CAD build for the part. Positions are in the model's coordinates, mm. Coordinates: 2 decimals unless noted, no trailing zeros. Loops run counter-clockwise (first coordinate to the right, second up) from the corner with the lowest first, then second, coordinate; pieces in that order, holes last. Notation, with made-up numbers: (-16, -5) -> (10, -5) arc R9 ccw to (10, 4) -> close; hole circle Ø4 at (71, 34). An arc over 180 degrees is marked (long way). Write item = value, one per line. Start each with the question number.
(1) Band-saw the part on A-A (z = 756.5). Write the cut outline in (x, y) (3 decimals).
(2) Drill centre lines: line 1 (Y direction, x = 3, z = 381) (1 decimal); line 2 (Y direction, x = 7.5, z = 381) (1 decimal); line 3 (X direction, y = -14, z = 315.5) (3 decimals). Where is each one in solid material? Low to high. Write a range as from..to.
(3) Band-saw the part on B-B (y = 0). Count the separate pieces of the cut face and the enclosed holes in it, and give its area (3 significant figures).
(4) Flat gauge pins, fed straight in: P1, Ø8, axis at y = 0, z = 177.8, coming from the +X side; P2, Ø11, axis at y = 0, z = 279.4, coming from the -X side (3 decimals); P3, Ø3, axis at x = -1, z = 454.5, coming from the +Y side (3 decimals); P4, Ø3, axis at x = 1, z = 246, coming from the -Y side (3 decimals). Where does each tip first touch, or does it go through?
```python
from build123d import *

# Parameters (mm, degrees)
F1_DEPTH = 914.4
F2_R     = 4.8895
F3_DEPTH = 31.751


with BuildPart() as f1:
    # F0 (on Top) → F1 (new body)
    with BuildSketch(Plane.XY):
        Polygon((3.175, -15.875), (15.875, -15.875), (15.875, 15.875), (3.175, 15.875), (3.175, 9.525), (-3.175, 9.525), (-3.175, 15.875), (-15.875, 15.875), (-15.875, -15.875), (-3.175, -15.875), (-3.175, -9.525), (3.175, -9.525), align=None)
    extrude(amount=F1_DEPTH)

    # F2 (on face) → F3 (cut, through all)
    with BuildSketch(Plane(origin=(-15.875, 0, 0), x_dir=(0, -1, 0), z_dir=(-1, 0, 0))):
        with Locations((0, 787.4)):
            Circle(F2_R)
        with Locations((0, 685.8)):
            Circle(F2_R)
        with Locations((0, 584.2)):
            Circle(F2_R)
        with Locations((0, 482.6)):
            Circle(F2_R)
        with Locations((0, 381)):
            Circle(F2_R)
        with Locations((0, 279.4)):
            Circle(F2_R)
        with Locations((0, 177.8)):
            Circle(F2_R)
        with Locations((0, 76.2)):
            Circle(F2_R)
    extrude(amount=-F3_DEPTH, mode=Mode.SUBTRACT)


solid = f1.part
```
Findings below:
q1.outline = (-15.875, -15.875) -> (-3.175, -15.875) -> (-3.175, -9.525) -> (3.175, -9.525) -> (3.175, -15.875) -> (15.875, -15.875) -> (15.875, 15.875) -> (3.175, 15.875) -> (3.175, 9.525) -> (-3.175, 9.525) -> (-3.175, 15.875) -> (-15.875, 15.875) -> close
q2.line_1 = -9.5..-4.9, 4.9..9.5
q2.line_2 = -15.9..-4.9, 4.9..15.9
q2.line_3 = -15.875..-3.175, 3.175..15.875
q3.separate_pieces = 9
q3.enclosed_holes = 0
q3.area = 26,500 mm²
q4.P1 = through
q4.P2 = -15.875
q4.P3 = 9.525
q4.P4 = -9.525
